```python
from build123d import *

# Parameters (mm, degrees)
F0_R     = 30
F0_R_2   = 19
F0_R_3   = 14
F1_DEPTH = 27
F2_DEPTH = 41
F3_R     = 2.5
F4_R     = 0.5
F5_SIZE  = 0.5


with BuildPart() as f1:
    # F0 (on Top) → F1 (new body)
    with BuildSketch(Plane.XY):
        Circle(F0_R)
        Circle(F0_R_2, mode=Mode.SUBTRACT)
        Circle(F0_R_2)
        Circle(F0_R_3, mode=Mode.SUBTRACT)
    extrude(amount=F1_DEPTH)

    # F0 (on Top) → F2 (join)
    with BuildSketch(Plane.XY):
        Circle(F0_R_2)
        Circle(F0_R_3, mode=Mode.SUBTRACT)
    extrude(amount=F2_DEPTH)

    # F3
    f3_edges = [f1.edges().sort_by_distance(p)[0] for p in [
        (-30, 0, 0),
        (-30, 0, 27),
    ]]
    fillet(f3_edges, radius=F3_R)

    # F4
    f4_edges = [f1.edges().sort_by_distance(p)[0] for p in [
        (-19, 0, 27),
        (-19, 0, 41),
    ]]
    fillet(f4_edges, radius=F4_R)

    # F5
    f5_edges = [f1.edges().sort_by_distance(p)[0] for p in [
        (-14, 0, 41),
        (-14, 0, 0),
    ]]
    chamfer(f5_edges, length=F5_SIZE)


solid = f1.part
```
Can you work these out from the model? Positions are in its coordinate system, mm. Coordinates: 2 decimals unless noted, no trailing zeros. Loops run counter-clockwise (first coordinate to the right, second up) from the corner with the lowest first, then second, coordinate; pieces in that order, holes last. Notation, with made-up numbers: (25.5, -6.75) -> (46.5, -6.75) arc R31 ccw to (46.5, 17.25) -> close; hole circle Ø7 at (22.25, 1.25). An arc over 180 degrees is marked (long way). Put each result on its own line as item: value. Start each with the question number.
Q1. I want a section at D-D (z = 22). Write out the boundary of the cut face in (x, y), plus the area to 3 significant figures.
Q2. I want a section at C-C (z = 34). Write out the boundary of the cut face in (x, y), plus the area to 3 significant figures.
Q3. I'm going to push flat-ended pins straight in: P1, Ø2, axis at y = 15, z = 13, coming from the +X side; P2, Ø4, axis at x = -8, z = 21, coming from the -Y side; P3, Ø10, axis at y = 4.5, z = 12.5, coming from the -X side; P4, Ø1.5, axis at x = -14, z = 6.5, coming from the -Y side. Where does each tip first touch, or does it pass through?
Q4. I want a section at A-A (y = 0). Write out the boundary of the cut face in (x, z).
Q5. If I drill on line 1 (Y direction, x = 0, z = 10); line 2 (Z direction, x = 20, y = 9.5); line 3 (X direction, y = 12.5, z = 36.5), over which ranges is the centre line in solid material (lowest first)? Write a range as [from, to].
Q6. Thinking about a two-plate mould opening in Y: for faces 1 (the face through (6, 19, 27)), 2 (the face through (12.932, -5.362, 20.22)), 3 (the face through (8.767, -16.856, 33.909)), which applies, pulls with the +Y half, pulls with the -Y half, needs draft (parallel to the pull), parting line crosses it, or undercut?
Taken from the geometry:
1. outline: circle Ø60 at (0, 0); hole circle Ø28 at (0, 0)
1. area: 2,210 mm2
2. outline: circle Ø38 at (0, 0); hole circle Ø28 at (0, 0)
2. area: 518 mm2
3. P1: stops at x = 26.53
3. P2: stops at y = -29.39
3. P3: stops at x = -30
3. P4: stops at y = -26.92
4. outline: (-30, 2.5) arc R2.5 ccw to (-27.5, 0) -> (-14.5, 0) -> (-14, 0.5) -> (-14, 40.5) -> (-14.5, 41) -> (-18.5, 41) arc R0.5 ccw to (-19, 40.5) -> (-19, 27.5) arc R0.5 cw to (-19.5, 27) -> (-27.5, 27) arc R2.5 ccw to (-30, 24.5) -> close; (14, 0.5) -> (14.5, 0) -> (27.5, 0) arc R2.5 ccw to (30, 2.5) -> (30, 24.5) arc R2.5 ccw to (27.5, 27) -> (19.5, 27) arc R0.5 cw to (19, 27.5) -> (19, 40.5) arc R0.5 ccw to (18.5, 41) -> (14.5, 41) -> (14, 40.5) -> close
5. line 1: y = [-30, -14], [14, 30]
5. line 2: z = [0, 27]
5. line 3: x = [-14.31, -6.3], [6.3, 14.31]
6. face 1: needs draft
6. face 2: undercut
6. face 3: parting line crosses it
